Verification items for the finished model (mm, model axes). Coordinates: 2 decimals unless noted, no trailing zeros. Loops run counter-clockwise (first coordinate to the right, second up) from the corner with the lowest first, then second, coordinate; pieces in that order, holes last. Notation, with made-up numbers: (38.25, 36.25) -> (97.25, 36.25) arc R27 cw to (97.25, 75.25) -> close; hole circle Ø11 at (2.25, -32.5). An arc over 180 degrees is marked (long way). Use CSV: the item, a comma, the result in double quotes. Start each with the question number.
```python
from build123d import *

# Parameters (mm, degrees)
F0_W     = 48
F0_H     = 1
F1_DEPTH = 1.5


with BuildPart() as f1:
    # F0 (on Right) → F1 (new body, symmetric)
    with BuildSketch(Plane.YZ):
        with Locations((-2.771254, -1.178571)):
            Rectangle(F0_W, F0_H)
        Polygon((-26.771254, -0.678571), (21.228746, -0.678571), (11.228746, 9.321429), (0.028746, 17.321429), (-11.771254, 22.421429), (-24.471254, 25.521429), (-40.371254, 28.121429), (-50.871254, 28.921429), (-60.371254, 27.521429), (-51.471254, 23.021429), (-43.771254, 17.321429), (-34.971254, 10.121429), (-30.571254, 5.881429), align=None)
    extrude(amount=F1_DEPTH, both=True)


solid = f1.part
```
1. Scan lines: line 1 (Z direction, x = -0.2, y = -46); line 2 (Z direction, x = 0.2, y = -18); line 3 (Y direction, x = 0.9, z = 2.5). Record each from-to range of solid material in increasing order.
2. Cross-section at C-C, the plane z = 15. Record the boundary of the cut face in (x, y), plus the area to 3 significant figures.
3. Cross-section at B-B, the plane y = -55. Record the boundary of the cut face in (x, z), plus the area to 3 significant figures.
4. Depth check by flat-ended pin: pin 1 (0.5 mm diameter, centred on x = 0.5, z = -1, fed in from -Y). Enter the tip coordinate at first touch or a pass-through.
5. Cross-section at A-A, the plane x = 0.2. Record the boundary of the cut face in (y, z), plus the area to 3 significant figures.
Solution:
1,line 1,"z = 18.97 to 28.55"
1,line 2,"z = -1.68 to 23.94"
1,line 3,"y = -28.61 to 18.05"
2,outline,"(-1.5, -40.93) -> (1.5, -40.93) -> (1.5, 3.28) -> (-1.5, 3.28) -> close"
2,area,"133 mm2"
3,outline,"(-1.5, 24.81) -> (1.5, 24.81) -> (1.5, 28.31) -> (-1.5, 28.31) -> close"
3,area,"10.5 mm2"
4,pin 1,"stops at y = -26.77"
5,outline,"(-60.37, 27.52) -> (-51.47, 23.02) -> (-43.77, 17.32) -> (-34.97, 10.12) -> (-30.57, 5.88) -> (-26.77, -0.68) -> (-26.77, -1.68) -> (21.23, -1.68) -> (21.23, -0.68) -> (11.23, 9.32) -> (0.03, 17.32) -> (-11.77, 22.42) -> (-24.47, 25.52) -> (-40.37, 28.12) -> (-50.87, 28.92) -> close"
5,area,"1,260 mm2"
